from build123d import *

# Parameters (mm, degrees)
EXTRUDE1_DEPTH          = 1155.7
SKETCH2_R               = 10.3124
EXTRUDE2_DEPTH          = 16.51
MIRROR2_COPY_1_SKETCH_R = 10.3124
MIRROR2_COPY_1_DEPTH    = 16.51


# Read off the part's stored shape, not the designer's step: 1515<1>
with BuildPart() as part:
    # Sketch1<2> → Extrude1 (new body)
    with BuildSketch(Plane(origin=(0, 0, 0), x_dir=(1, 0, 0), z_dir=(0, 1, 0))):
        Polygon((-6.7564, 4.364749804), (-6.7564, -4.364749804), (-14.986, -12.594349804), (-14.986, -4.064), (-19.05, -4.064), (-19.05, -19.05), (-4.064, -19.05), (-4.064, -14.986), (-13.067127258, -14.986), (-4.837527258, -6.7564), (4.837527258, -6.7564), (13.067127258, -14.986), (4.064, -14.986), (4.064, -19.05), (19.05, -19.05), (19.05, -4.064), (14.986, -4.064), (14.986, -12.594349804), (6.7564, -4.364749804), (6.7564, 4.364749804), (14.986, 12.594349804), (14.986, 4.064), (19.05, 4.064), (19.05, 19.05), (4.064, 19.05), (4.064, 14.986), (13.067127258, 14.986), (4.837527258, 6.7564), (-4.837527258, 6.7564), (-13.067127258, 14.986), (-4.064, 14.986), (-4.064, 19.05), (-19.05, 19.05), (-19.05, 4.064), (-14.986, 4.064), (-14.986, 12.594349804), align=None)
    extrude(amount=EXTRUDE1_DEPTH)

    # Sketch2 → Extrude2 (cut)
    with BuildSketch(Plane.ZY.offset(19.05)):
        with Locations(Location((0, 1133.983, 0), (0, 0, 310.932724574))):
            Circle(SKETCH2_R)
    extrude2 = extrude(amount=-EXTRUDE2_DEPTH, mode=Mode.SUBTRACT)

    # Mirror1: Extrude2 across plane
    add(extrude2.mirror(Plane(origin=(0, 0, 0), x_dir=(0, 0, 1), z_dir=(1, 0, 0))), mode=Mode.SUBTRACT)

    # Mirror2: Extrude2 across plane
    add(extrude2.mirror(Plane(origin=(0, 577.85, 0), x_dir=(0, 0, 1), z_dir=(0, -1, 0))), mode=Mode.SUBTRACT)

    # Mirror2 copy 1 sketch → Mirror2 copy 1 (cut)
    with BuildSketch(Plane(origin=(19.05, 1155.7, 0), x_dir=(0, 0, 1), z_dir=(1, 0, 0))):
        with Locations(Location((0, 1133.983, 0), (0, 0, 310.932724574))):
            Circle(MIRROR2_COPY_1_SKETCH_R)
    extrude(amount=-MIRROR2_COPY_1_DEPTH, mode=Mode.SUBTRACT)


solid = part.part
The model under review builds one solid part; all positions refer to its coordinate system, in mm. A direction names the side the tool comes from. Give positions to 0.01 mm unless a question says otherwise; leave off trailing zeros. One line per question, with ' | ' between items. Start each with the question number.
Item 1: For pin 1 (2.5 mm diameter, centred on y = 1147, z = -1, fed in from +X); pin 2 (11 mm diameter, centred on y = 1133.5, z = -1.5, fed in from -X); pin 3 (7 mm diameter, centred on y = 18.5, z = -1, fed in from +X), all flat-tipped, find the tip position at first contact; note any pin that passes through.
Item 2: Wall thickness on line 1 (Z direction, x = 5, y = 697.5); line 2 (Y direction, x = -5.25, z = 0); line 3 (Z direction, x = 4.5, y = 212): over which ranges is each line inside the solid? List them lowest first. Write a range as from..to.
Item 3: For faces 1 (the cylindrical face through (6.83, 1142.06, -6.41)), 2 (the flat face through (0, 1155.7, 0)), 3 (the cylindrical face through (-6.83, 13.64, -6.41)), list the 3-axis set-ups (+Z, -Z, +X, -X, +Y, -Y) from which the entire face can be reached by the end or side of a thin tool; tool diameter is ignored.
Results found:
1) pin 1: stops at x = 6.76 | pin 2: stops at x = -2.54 | pin 3: stops at x = 2.54
2) line 1: z = -19.05..-14.99, -6.92..6.92, 14.99..19.05 | line 2: y = 0..11.4, 32.03..1123.67, 1144.3..1155.7 | line 3: z = -19.05..-14.99, -6.76..6.76, 14.99..19.05
3) face 1: +X | face 2: +Z, -Z, +X, -X, +Y | face 3: -X
